Geometry check sheet. Reference: the model listing, model coordinates, mm. Round coordinates to 2 decimals unless told otherwise and drop trailing zeros. Write each loop counter-clockwise with the first axis right and the second up, starting at its lowest first coordinate (ties: lowest second). Pieces come first, ordered by that corner, then holes. Notation, with made-up numbers: M -25.75,-3.5 L 29.25,-3.5 A25 cw 29.25,9.5 Z; hole C 46.5,86 d10. An arc over 180 degrees is marked long. One line per item, written item: value. Start each with the question number.
1. Section check C-C (z = 59.5). Record the boundary of the cut face in (x, y).
2. Section check B-B (x = 5). Record the boundary of the cut face in (y, z).
3. Scan lines: probe 1 along X at (y, z) = (-3.25, 35); probe 2 along X at (y, z) = (4, 20); probe 3 along Y at (x, z) = (-5.25, 80.5). Record each from-to range of solid material in increasing order. Write a range as [from, to].
4. Section check A-A (y = -3.5). Record the boundary of the cut face in (x, z).
from build123d import *

# Parameters (mm, degrees)
BOSS_EXTRUDE1_DEPTH = 101.6
CHAMFER1_SIZE       = 0.254


with BuildPart() as part:
    # Sketch1 → Boss-Extrude1 (new body)
    with BuildSketch(Plane(origin=(0, 0, 0), x_dir=(-1, 0, 0), z_dir=(0, 0, -1))):
        Polygon((3.666174209, 6.35), (-3.666174209, 6.35), (-7.332348419, 0), (-3.666174209, -6.35), (3.666174209, -6.35), (7.332348419, 0), align=None)
    extrude(amount=-BOSS_EXTRUDE1_DEPTH)

    # Chamfer1
    chamfer1_edges = [part.edges().sort_by_distance(p)[0] for p in [
        (5.499261314, 3.175, 101.6),
        (5.499261314, -3.175, 101.6),
        (0, -6.35, 101.6),
        (-5.499261314, -3.175, 101.6),
        (-5.499261314, 3.175, 101.6),
        (-5.499261314, -3.175, 0),
        (0, -6.35, 0),
        (5.499261314, -3.175, 0),
        (5.499261314, 3.175, 0),
        (0, 6.35, 0),
        (-5.499261314, 3.175, 0),
        (0, 6.35, 101.6),
    ]]
    chamfer(chamfer1_edges, length=CHAMFER1_SIZE)


solid = part.part
Result sheet:
1. outline: M -7.33,0 L -3.67,-6.35 L 3.67,-6.35 L 7.33,0 L 3.67,6.35 L -3.67,6.35 Z
2. outline: M -4.04,0.25 L -3.53,0 L 3.53,0 L 4.04,0.25 L 4.04,101.35 L 3.53,101.6 L -3.53,101.6 L -4.04,101.35 Z
3. probe 1: x = [-5.46, 5.46]
3. probe 2: x = [-5.02, 5.02]
3. probe 3: y = [-3.61, 3.61]
4. outline: M -5.31,0.25 L -5.02,0 L 5.02,0 L 5.31,0.25 L 5.31,101.35 L 5.02,101.6 L -5.02,101.6 L -5.31,101.35 Z
